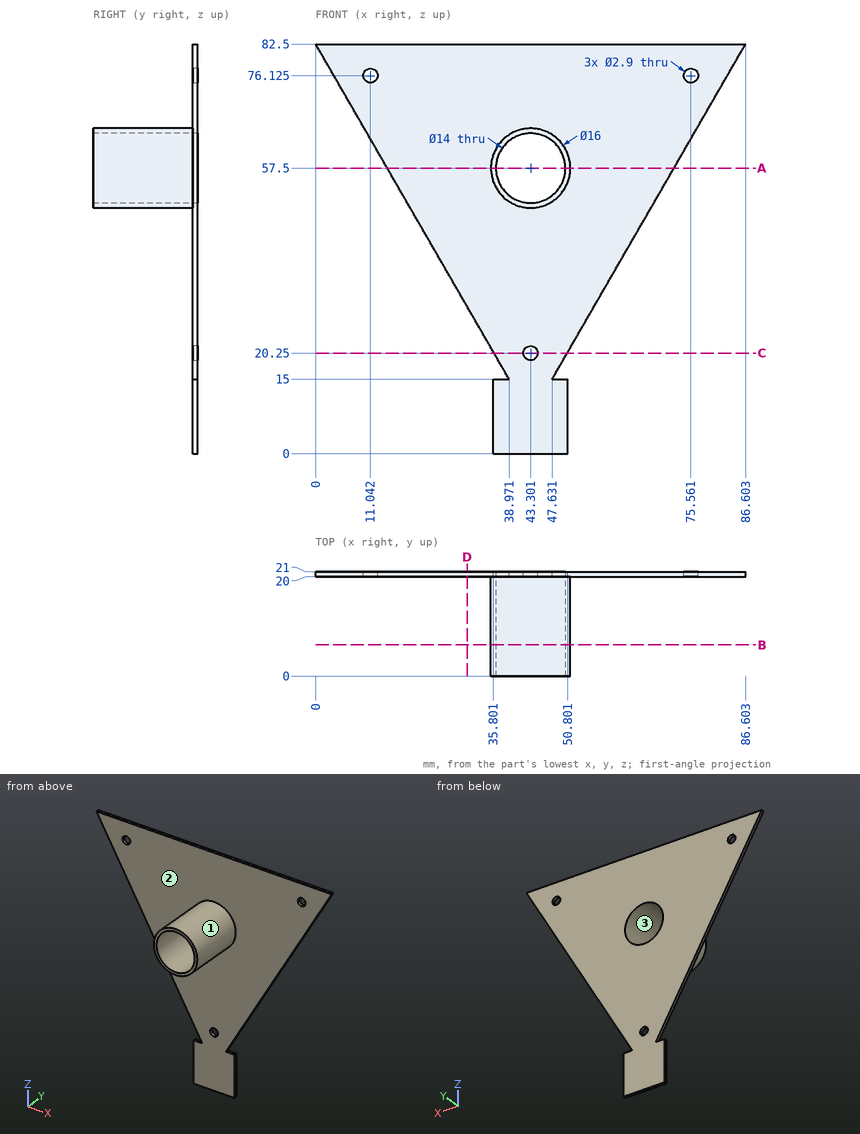
Could you check a few things on this drawing? It's one solid part, dimensions in mm from its lowest x, y, z. Coordinates: 2 decimals unless noted, no trailing zeros. Write each loop counter-clockwise with the first axis right and the second up, starting at its lowest first coordinate (ties: lowest second). Pieces come first, ordered by that corner, then holes.
Q1. For P1, Ø2, axis at y = 14, z = 68, coming from the +X side; P2, Ø0.5, axis at y = 20.5, z = 10, coming from the -X side; P3, Ø5, axis at x = 57.5, z = 40.5, coming from the -Y side; P4, Ø1.1, axis at y = 20.5, z = 5.5, coming from the +X side, each with a flat end and sliding along its axis, tell me the tip position at first contact or that it passes through.
Results found:
P1: passes through
P2: stops at x = 35.8
P3: stops at y = 20
P4: stops at x = 50.8
Q2. Please list where these lines run through material, in increasing order: L1, parallel to X at y = 6, z = 57.5; L2, parallel to Y at x = 26.5, z = 46; L3, parallel to Z at x = 46, y = 17.5.
Results found:
L1: x = 35.3 to 36.3, 50.3 to 51.3
L2: y = 20 to 21
L3: z = 49.97 to 51.04, 63.96 to 65.03
Q3. Imagine slicing it at B-B, the plane y = 6.25. List the corners of the cut face in (x, z) for me.
Results found:
outline: circle Ø16 at (43.3, 57.5); hole circle Ø14 at (43.3, 57.5)
Q4. Imagine slicing it at A-A, the plane z = 57.5. List the corners of the cut face in (x, y) for me.
Results found:
outline: (14.43, 20) - (35.3, 20) - (35.3, 0) - (36.3, 0) - (36.3, 21) - (14.43, 21) - close; (50.3, 0) - (51.3, 0) - (51.3, 20) - (72.17, 20) - (72.17, 21) - (50.3, 21) - close
Q5. Imagine slicing it at C-C, the plane z = 20.25. List the corners of the cut face in (x, y) for me, plus the area to 3 significant figures.
Results found:
outline: (35.94, 20) - (41.85, 20) - (41.85, 21) - (35.94, 21) - close; (44.75, 20) - (50.66, 20) - (50.66, 21) - (44.75, 21) - close
area: 11.8 mm2
Q6. Imagine slicing it at D-D, the plane x = 30.5. List the corners of the cut face in (y, z) for me.
Results found:
outline: (20, 29.67) - (21, 29.67) - (21, 82.5) - (20, 82.5) - close
Q7. If we mould it in two halves opening along X, with no side actions, what happens to the marked faces 1, 2 and 3? For each: +X half, -X half, draft (parallel to the pull), parting line (faces both ways), or undercut.
Results found:
face 1: parting line
face 2: draft
face 3: undercut
